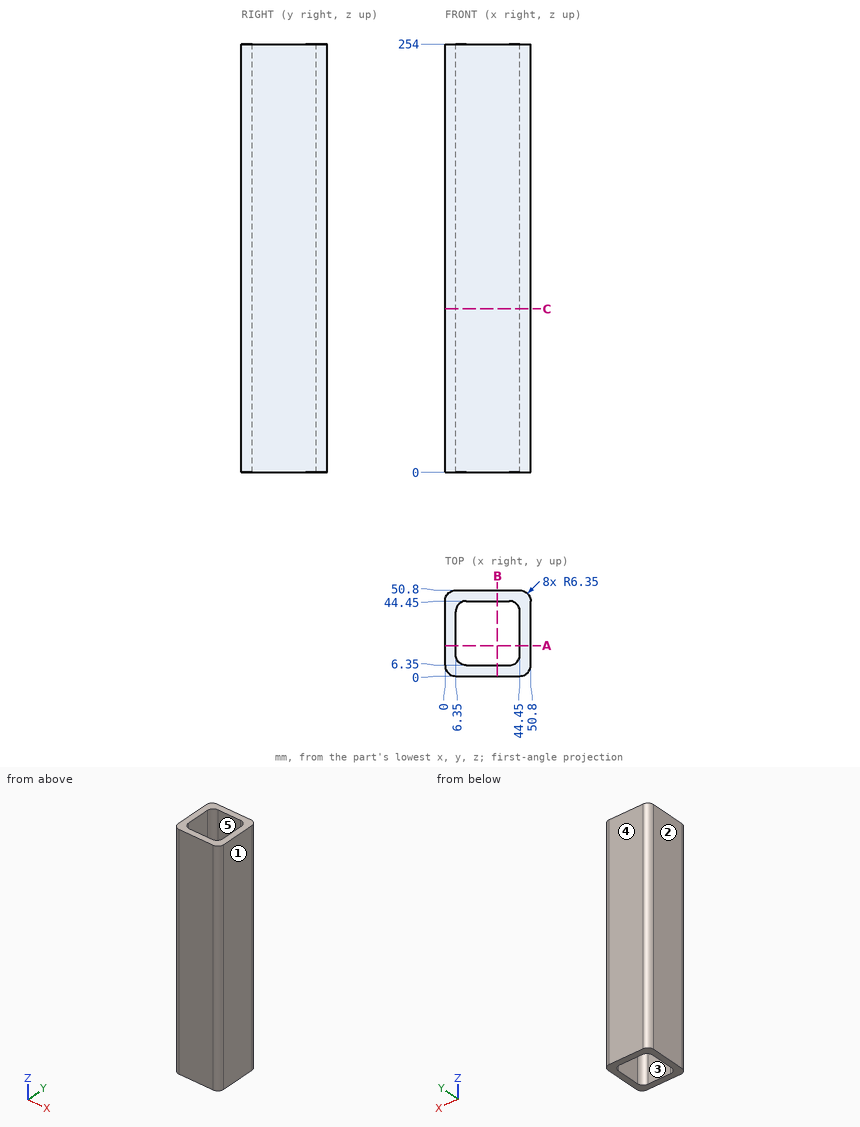
The drawing under review shows one solid part. Ordinate dimensions are in mm from its lowest x, y, z. A direction names the side the tool comes from. Coordinates: 2 decimals unless noted, no trailing zeros. Order: outer loops, then holes, each group sorted by start corner. A loop starts at its lowest first (then second) coordinate and runs counter-clockwise, first axis right, second up. Notation, with made-up numbers: (9.5, 29) -> (21.5, 29) arc R8 ccw to (21.5, 36) -> close; hole circle Ø8 at (75, 8.25). An arc over 180 degrees is marked (long way). Answer in a Markdown table with one row per item. Add a question column.
Item 1: We need section A-A on y = 18. Write out the cut boundary in (x, z), plus the area to 3 significant figures.
Item 2: Machinability: for the marked faces 4 and 5, which of the approach directions +Z, -Z, +X, -X, +Y, -Y give a long, thin tool a straight path to every point of the face, cutting with its end or side? Answer none if there is none.
Item 3: We need section C-C on z = 97. Write out the cut boundary in (x, y).
Item 4: Mouldability with a two-part tool opening along X and no side actions: class the marked faces 1, 2 and 3 as +X half, -X half, draft (parallel to the pull), parting line (faces both ways), or undercut.
Item 5: To check wall thickness, follow probe 1 along Y at (x, z) = (37, 184); probe 2 along Y at (x, z) = (45, 189). State the ranges of each line that lie inside material, in increasing order.
Item 6: Clearance check with a flat-ended pin moving along its axis: pin 1 (20.5 mm diameter, centred on y = 24.5, z = 146, fed in from -X). State where the tip first meets the part, or that it passes through.
Final values:
| question | item | result |
|---|---|---|
| 1 | outline | (0, 0) -> (6.35, 0) -> (6.35, 254) -> (0, 254) -> close; (44.45, 0) -> (50.8, 0) -> (50.8, 254) -> (44.45, 254) -> close |
| 1 | area | 3,230 mm2 |
| 2 | face 4 | +Z, -Z, +X, -X, +Y |
| 2 | face 5 | +Z, -Z |
| 3 | outline | (0, 6.35) arc R6.35 ccw to (6.35, 0) -> (44.45, 0) arc R6.35 ccw to (50.8, 6.35) -> (50.8, 44.45) arc R6.35 ccw to (44.45, 50.8) -> (6.35, 50.8) arc R6.35 ccw to (0, 44.45) -> close; hole (6.35, 12.7) arc R6.35 ccw to (12.7, 6.35) -> (38.1, 6.35) arc R6.35 ccw to (44.45, 12.7) -> (44.45, 38.1) arc R6.35 ccw to (38.1, 44.45) -> (12.7, 44.45) arc R6.35 ccw to (6.35, 38.1) -> close |
| 4 | face 1 | +X half |
| 4 | face 2 | -X half |
| 4 | face 3 | undercut |
| 5 | probe 1 | y = 0 to 6.35, 44.45 to 50.8 |
| 5 | probe 2 | y = 0.02 to 50.78 |
| 6 | pin 1 | stops at x = 0 |
